Geometry: final body of the model. Coordinates: model frame, mm. A direction names the side the tool comes from. Give positions to 0.01 mm unless a question says otherwise; leave off trailing zeros. Write each loop counter-clockwise with the first axis right and the second up, starting at its lowest first coordinate (ties: lowest second). Pieces come first, ordered by that corner, then holes.
Q1. Draft query along X for faces 1 (the face through (-40.018, 7, 30)), 2 (the face through (-112, 0, 29.5)), 3 (the face through (-45.018, 7, 38)). Return one class per face: pulls with the +X half, pulls with the -X half, needs draft (parallel to the pull), parting line crosses it, or undercut.
Q2. Cut plane B-B on x = 52.5. Return the cut outline in (y, z), plus the area to 4 significant figures.
Q3. Reachability of faces 4 (the face through (98.469, 8.642, -3.944)), 5 (the face through (-27.518, 7, 38)), 6 (the face through (-112, 0, 5.5)), 7 (the face through (-24.5, 0, 15)), 8 (the face through (-35, 7, 1)) from +Z, -Z, +X, -X, +Y, -Y: full face, straight path, thin tool, end or side. Return the list, or none.
Q4. Cut plane A-A on z = 13.5. Return the cut outline in (x, y).
Q5. Pin query (flat end, axial travel): pin 1 (6 mm diameter, centred on y = 2, z = 11, fed in from -X); pin 2 (10.5 mm diameter, centred on x = -17, y = 0, fed in from -Z); pin 3 (3.5 mm diameter, centred on x = -43, z = 39, fed in from +Y); pin 4 (12 mm diameter, centred on x = 97, y = -8.5, fed in from -Z). Return the tip coordinate at first contact, or that it passes through.
Q6. Cut plane C-C on x = 107.5. Return the cut outline in (y, z), plus the area to 4 significant figures.
Q7. Line query: L1, parallel to Y at x = 52.5, z = 15; L2, parallel to Z at x = -112.5, y = -4; L3, parallel to X at y = 0, z = 7.5. Output: solid intervals per line, ascending.
Q8. Cut plane D-D on x = 20.5. Return the cut outline in (y, z).
```python
from build123d import *

# Parameters (mm, degrees)
F1_DEPTH  = 35
F3_D      = 6.5
F3_DEPTH  = 35
F3_TIP    = 1.9527970118
F4_D      = 6.5
F4_DEPTH  = 35
F4_TIP    = 1.9527970118
F6_W      = 24
F6_H      = 24
F7_DEPTH  = 25.5
F9_DEPTH  = 8
F11_DEPTH = 8
F12_W     = 20.5
F12_H     = 20.5
F13_DEPTH = 100
F14_W     = 10.5
F14_H     = 6.5
F16_DEPTH = 34
F15_W     = 3
F15_H     = 6.5
F17_DEPTH = 6


with BuildPart() as f1:
    # F0 (on Top) → F1 (new body)
    with BuildSketch(Plane.XY):
        Polygon((90, -17.5), (125, 17.5), (-125, 17.5), (-125, -17.5), align=None)
    extrude(amount=F1_DEPTH)

    # F3
    with Locations(Plane.XY.offset(35)):
        with Locations((-70, 0)):
            Hole(F3_D / 2, depth=F3_DEPTH)
            with Locations((0, 0, -(F3_DEPTH + F3_TIP / 2))):  # 118° drill point
                Cone(0, F3_D / 2, F3_TIP, mode=Mode.SUBTRACT)

    # F4
    with Locations(Plane.XY.offset(35)):
        with Locations((52.5, 0)):
            Hole(F4_D / 2, depth=F4_DEPTH)
            with Locations((0, 0, -(F4_DEPTH + F4_TIP / 2))):  # 118° drill point
                Cone(0, F4_D / 2, F4_TIP, mode=Mode.SUBTRACT)

    # F6 (on face) → F7 (cut)
    with BuildSketch(Plane(origin=(-125, 0, 0), x_dir=(0, -1, 0), z_dir=(-1, 0, 0))):
        with Locations((0, 17.5)):
            Rectangle(F6_W, F6_H)
    extrude(amount=-F7_DEPTH, mode=Mode.SUBTRACT)

    # F8 (on face) → F9 (join)
    with BuildSketch(Plane(origin=(0, 0, 0), x_dir=(1, 0, 0), z_dir=(0, 0, -1))):
        with BuildLine():
            Line((116.3388347648, -8.8388347648), (98.6611652352, 8.8388347648))
            ThreePointArc((98.6611652352, 8.8388347648), (98.6611652352, -8.8388347648), (116.3388347648, -8.8388347648))
        make_face()
    extrude(amount=F9_DEPTH)

    # F10 (on face) → F11 (join)
    with BuildSketch(Plane(origin=(0, 0, 0), x_dir=(1, 0, 0), z_dir=(0, 0, -1))):
        with BuildLine():
            ThreePointArc((-125, -12.5), (-116.1611652352, -8.8388347648), (-112.5, 0))
            ThreePointArc((-112.5, 0), (-116.1611652352, 8.8388347648), (-125, 12.5))
            Line((-125, 12.5), (-125, -12.5))
        make_face()
    extrude(amount=F11_DEPTH)

    # F12 (on face) → F13 (cut)
    with BuildSketch(Plane(origin=(0, 17.5, 0), x_dir=(-1, 0, 0), z_dir=(0, 1, 0))):
        with Locations((34.75, 14.75)):
            Rectangle(F12_W, F12_H)
    extrude(amount=-F13_DEPTH, mode=Mode.SUBTRACT)

    # F14 (on face) → F16 (cut)
    with BuildSketch(Plane.XY.offset(35)):
        with Locations((-34.7681139037, 6.6779768765)):
            Rectangle(F14_W, F14_H)
    extrude(amount=-F16_DEPTH, mode=Mode.SUBTRACT)

    # F15 (on face) → F17 (join)
    with BuildSketch(Plane.XY.offset(35)):
        with Locations((-43.5181139037, 6.6779768765)):
            Rectangle(F15_W, F15_H)
        with Locations((-26.0181139037, 6.6779768765)):
            Rectangle(F15_W, F15_H)
    extrude(amount=F17_DEPTH)


solid = f1.part
```
Data:
1. face 1: undercut
1. face 2: needs draft
1. face 3: pulls with the -X half
2. outline: (-17.5, 0) - (-3.25, 0) - (-3.25, 35) - (-17.5, 35) - close; (3.25, 0) - (17.5, 0) - (17.5, 35) - (3.25, 35) - close
2. area: 997.5 mm2
3. face 4: -Z
3. face 5: +Z, +Y, -Y
3. face 6: -X
3. face 7: +Y, -Y
3. face 8: +Z
4. outline: (-125, -17.5) - (-45, -17.5) - (-45, 17.5) - (-125, 17.5) - (-125, 12) - (-99.5, 12) - (-99.5, -12) - (-125, -12) - close; (-24.5, -17.5) - (90, -17.5) - (125, 17.5) - (-24.5, 17.5) - close; hole circle Ø6.5 at (-70, 0); hole circle Ø6.5 at (52.5, 0)
5. pin 1: stops at x = -99.5
5. pin 2: stops at z = 0
5. pin 3: stops at y = 9.93
5. pin 4: stops at z = -8
6. outline: (0, -8) - (12.5, -8) - (12.5, 0) - (17.5, 0) - (17.5, 35) - (0, 35) - close
6. area: 712.5 mm2
7. L1: y = -17.5 to -3.25, 3.25 to 17.5
7. L2: z = 0 to 5.5, 29.5 to 35
7. L3: x = -99.5 to -73.25, -66.75 to -45, -24.5 to 49.25, 55.75 to 107.5
8. outline: (-17.5, 0) - (17.5, 0) - (17.5, 35) - (-17.5, 35) - close
